Part print with two shaded views. Sizes in mm from the minimum x, y, z corner. A direction names the side the tool comes from. Give positions to 0.01 mm unless a question says otherwise; leave off trailing zeros. Write each loop counter-clockwise with the first axis right and the second up, starting at its lowest first coordinate (ties: lowest second). Pieces come first, ordered by that corner, then holes. Notation, with made-up numbers: (-17.75, -34.75) - (-8.75, -34.75) arc R28 ccw to (-8.75, 1.25) - close; hole circle Ø7 at (1.25, 20.5). An arc over 180 degrees is marked (long way). Answer as a JSON object with one key per item and string values. Group by question number.
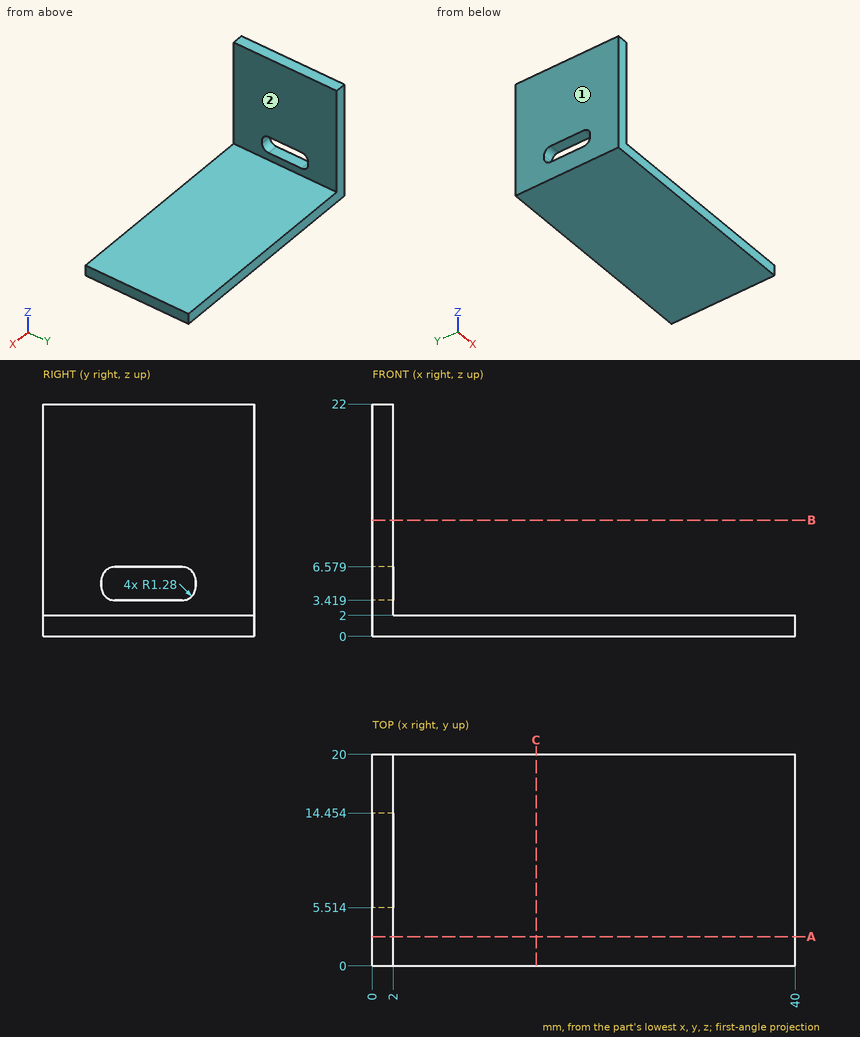
1) Drop flat-ended pins along their axis: P1, Ø1.5, axis at y = 2.5, z = 8.5, coming from the +X side; P2, Ø5, axis at x = 12.5, y = 13.5, coming from the +Z side. Give the stop position or say it passes through.
2) Which spindle directions (+Z, -Z, +X, -X, +Y, -Y) get a long thin tool onto all of the face, cutting with end or side? Do the marked faces 1 and 2. Say none if no direction does.
3) Saw through at B-B (z = 11). List the corners of the cut face in (x, y).
4) Drill centre line: line 1 along Z through (x, y) = (31.5, 15.75). Where is it in solid material? Low to high. Write a range as from..to.
5) Saw through at A-A (y = 2.75). List the corners of the cut face in (x, z), and give its area (3 significant figures).
6) Saw through at C-C (x = 15.5). List the corners of the cut face in (y, z), and give its area (3 significant figures).
Checks:
{
 "1": {"P1": "x = 2", "P2": "z = 2"},
 "2": {"face 1": "+Z, -Z, -X, +Y, -Y", "face 2": "+Z, +X, +Y, -Y"},
 "3": {"outline": "(0, 0) - (2, 0) - (2, 20) - (0, 20) - close"},
 "4": {"line 1": "0..2"},
 "5": {"outline": "(0, 0) - (40, 0) - (40, 2) - (2, 2) - (2, 22) - (0, 22) - close", "area": "120 mm2"},
 "6": {"outline": "(0, 0) - (20, 0) - (20, 2) - (0, 2) - close", "area": "40.0 mm2"}
}
